Part print with two shaded views. Sizes in mm from the minimum x, y, z corner. Give positions to 0.01 mm unless a question says otherwise; leave off trailing zeros. Write each loop counter-clockwise with the first axis right and the second up, starting at its lowest first coordinate (ties: lowest second). Pieces come first, ordered by that corner, then holes. Notation, with made-up numbers: (3, 73) - (56, 73) arc R19 cw to (56, 98) - close; hole circle Ø10 at (-22.5, 14). An arc over 180 degrees is marked (long way). One line per item, written item: value. Start each with the question number.
(1) Cut at A-A, the plane y = 50.5. List the corners of the cut face in (x, z).
(2) Cut at B-B, the plane z = 16. List the corners of the cut face in (x, y), and give its area (3 significant figures).
(3) Probe L1, parallel to Y at x = 4, z = 37.5; L2, parallel to X at y = 7, z = 37; L3, parallel to X at y = 28, z = 28. List the from-to ranges inside material, lowest first.
(4) Drop flat-ended pins along their axis: P1, Ø1, axis at x = 19, y = 14.5, coming from the +Z side; P2, Ø3, axis at y = 12.5, z = 43.5, coming from the +X side; P3, Ø1.5, axis at y = 48, z = 18, coming from the +X side. Give the stop position or say it passes through.
(5) Cut at D-D, the plane y = 28.5. List the corners of the cut face in (x, z), and give its area (3 significant figures).
(6) Cut at C-C, the plane x = 3.5. List the corners of the cut face in (y, z), and give its area (3 significant figures).
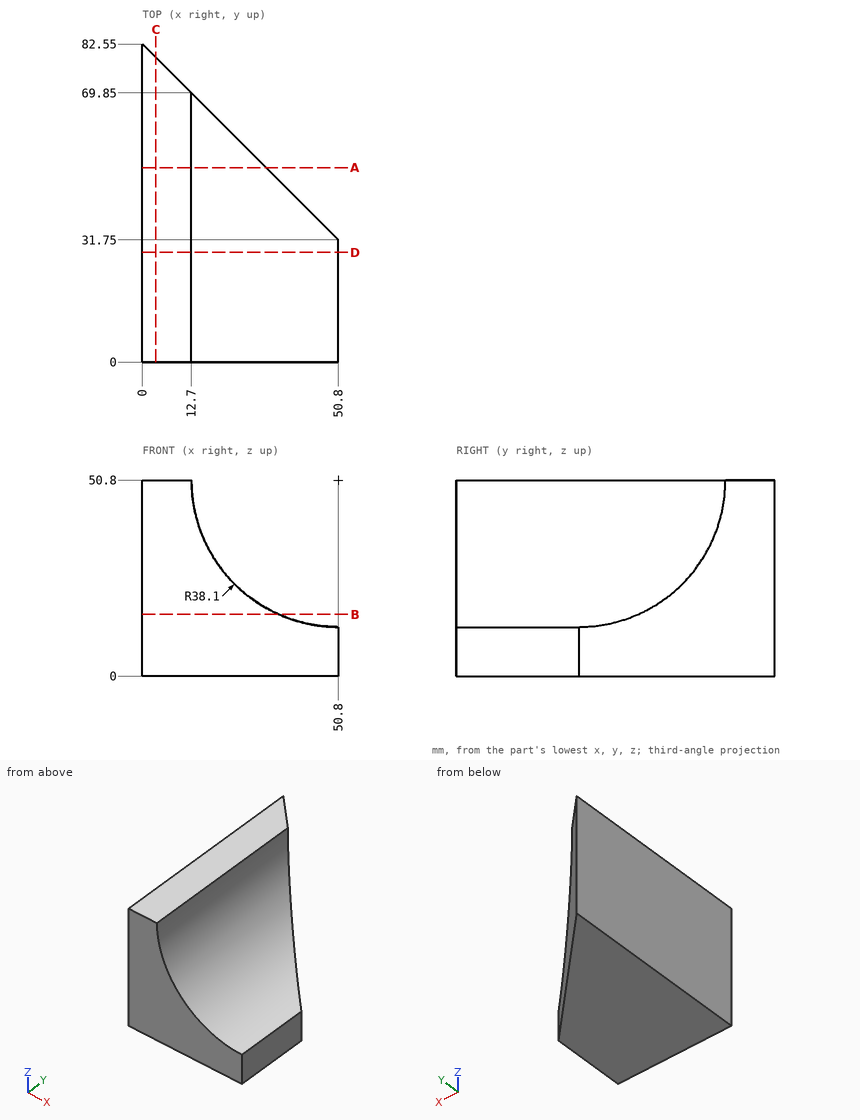
Answers follow:
1. outline: (0, 0) - (32.05, 0) - (32.05, 17.63) arc R38.1 cw to (12.7, 50.8) - (0, 50.8) - close
2. outline: (0, 0) - (35.29, 0) - (35.29, 47.26) - (0, 82.55) - close
2. area: 2,290 mm²
3. L1: y = 0 to 78.55
3. L2: x = 0 to 15.29
3. L3: x = 0 to 20.28
4. P1: stops at z = 30.59
4. P2: stops at x = 13.73
4. P3: stops at x = 32.74
5. outline: (0, 0) - (50.8, 0) - (50.8, 12.7) arc R38.1 cw to (12.7, 50.8) - (0, 50.8) - close
5. area: 1,440 mm²
6. outline: (0, 0) - (79.05, 0) - (79.05, 50.8) - (0, 50.8) - close
6. area: 4,020 mm²
